Autodesk Inventor part; units mm, degrees
ref_plane "YZ Plane" through (0, 0, 0) normal (1, 0, 0) x (0, 1, 0)
ref_plane "XZ Plane" through (0, 0, 0) normal (0, 1, 0) x (-1, 0, 0)
ref_plane "XY Plane" through (0, 0, 0) normal (0, 0, 1) x (1, 0, 0)
sketch "Esboço1" plane through (0, 0, 0) normal (1, 0, 0) x (0, 1, 0)
  line L0 (0, 0) -> (0, -144)
  line L1 (0, -144) -> (52, -144)
  line L2 (52, -144) -> (52, -122)
  line L3 (52, -122) -> (16, -122)
  line L4 (0, 0) -> (38, 0)
  line L5 (38, 0) -> (52, 0)
  line L6 (16, -122) -> (16, -26)
  line L7 (16, -26) -> (52, -26)
  line L8 (52, -26) -> (52, -16)
  line L9 (52, -16) -> (38, 0)
  dimension "d0" = 144
  dimension "d1" = 52
  dimension "d2" = 22
  dimension "d3" = 36
  dimension "d8" = 38
  dimension "d10" = 96
  dimension "d12" = 10
extrude "Extrusão1" add sketch "Esboço1" against normal blind 64
sketch "Esboço2" plane through (0, 0, -144) normal (0, 0, -1) x (-1, 0, 0)
  line L0 (0, 0) -> (16, 0)
  line L1 (0, 0) -> (64, 0)
  line L2 (16, 0) -> (16, 7)
  line L3 (16, 7) -> (24, 7)
  line L4 (24, 7) -> (24, 16)
  line L5 (24, 16) -> (40, 16)
  line L6 (0, 16) -> (64, 16)
  line L7 (40, 16) -> (40, 7)
  line L8 (40, 7) -> (48, 7)
  line L9 (48, 7) -> (48, 0)
  dimension "d15" = 16
  dimension "d16" = 7
  dimension "d20" = 16
  dimension "d21" = 9
  dimension "d22" = 8
extrude "Extrusão2" cut sketch "Esboço2" against normal blind 144
sketch "Esboço3" plane through (0, 0, -144) normal (0, 0, -1) x (-1, 0, 0)
  point P0 (0, 0)
sketch "Esboço5" plane through (0, 0, -144) normal (0, 0, -1) x (-1, 0, 0)
  line L0 (48, 0) -> (64, 0)
  line L1 (0, 52) -> (64, 52)
  line L2 (64, 52) -> (64, 0)
  line L3 (40, 16) -> (64, 16)
  line L4 (24, 16) -> (40, 16)
  circle A0 centre (32, 36) radius 16
  line L5 (46.3807, 43.0139) -> (59.5563, 16)
  line L6 (17.6193, 43.0139) -> (4.4437, 16)
  line L7 (0, 0) -> (0, 52)
  line L8 (0, 0) -> (0, 16)
  line L9 (0, 16) -> (4.4437, 16)
  line L10 (0, 16) -> (24, 16)
  line L11 (59.5563, 16) -> (64, 16)
  line L12 (64, 16) -> (64, 0)
  point P0 (32, 52)
extrude "Extrusão3" cut sketch "Esboço5" against normal blind 22 contours L1 A0 L6 L9 L7 | L1 L2 L3 L5 A0
sketch "Esboço6" plane through (0, 0, -144) normal (0, 0, -1) x (-1, 0, 0)
  line L0 (24, 16) -> (40, 16)
  line L1 (32, 16) -> (32, 36)
  point P0 (0, 0)
  dimension "d49" = 20
hole "Furo1" at (-32, 36, -144) direction (0, 0, 1) diameter 13.835 depth 22
sketch "Esboço7" plane through (-64, 0, -144) normal (0, -1, 0) x (1, 0, 0)
  line L0 (0, 144) -> (0, 128)
  line L1 (10, 108) -> (10, 36)
  line L2 (54, 108) -> (54, 36)
  point P0 (64, 144)
  dimension "d59" = 72
  dimension "d61" = 72
hole "Furo2" at (-10, 0, -36) at (-10, 0, -108) at (-54, 0, -108) at (-54, 0, -36) direction (0, 1, 0) diameter 4.917 depth 12 tip angle 118
properties part number "morsa_body" material "Iron, Cast"
Geometry: final body of the model. Coordinates: model frame, mm. A direction names the side the tool comes from. Coordinates: 2 decimals unless noted, no trailing zeros. Order: outer loops, then holes, each group sorted by start corner. A loop starts at its lowest first (then second) coordinate and runs counter-clockwise, first axis right, second up. Notation, with made-up numbers: M 86.25,60 L 107.25,60 A19 cw 107.25,92 Z; hole C 28.5,38 d6. An arc over 180 degrees is marked long. Answer in a Markdown table with one row per item. Add a question column.
Q1. Contact query for flat-ended pins moving along their axis: P1, Ø12.5, axis at x = -32, y = 36, coming from the -Z side; P2, Ø2, axis at x = -17, z = -67, coming from the +Y side; P3, Ø4, axis at x = -20, z = -82, coming from the -Y side. Output: stop coordinate, or through.
Q2. Section query A-A on y = 5. Return the cut outline in (x, z), and give its area (3 significant figures).
Q3. Line query: L1, parallel to X at y = 7.75, z = -36; L2, parallel to Z at x = -10, y = 7; L3, parallel to Z at x = -32.5, y = 23. Output: solid intervals per line, ascending.
Q4. Mould query, pull axis Z, two halves, no side actions, for faces 6 (the flat face through (-40, 12, -73)), 7 (the cylindrical face through (-53.06, 6.08, -110.27)), 8 (the flat face through (-32, 45, -8)). Classes: released by +Z, released by -Z, zero draft, split by the parting line, or undercut.
Q5. Reachability of faces 1 (the cylindrical face through (-10.738, 6.084, -110.345)), 2 (the flat face through (-11.124, 29.696, -133.154)), 3 (the flat face through (-8, 0, -71)), 4 (the flat face through (-52.876, 29.696, -133.154)), 5 (the flat face through (-48, 4, -73)) from +Z, -Z, +X, -X, +Y, -Y: full face, straight path, thin tool, end or side. Return the list, or none.
Q6. Section query B-B on z = -60.5. Return the cut outline in (x, y).
Q7. Section query C-C on x = -32. Return the cut outline in (y, z).
Q8. Section query D-D on z = -125. Return the cut outline in (x, y) (1 decimal).
Completed:
| question | item | result |
|---|---|---|
| 1 | P1 | stops at z = -26 |
| 1 | P2 | stops at y = 16 |
| 1 | P3 | stops at y = 7 |
| 2 | outline | M -64,-144 L -48,-144 L -48,0 L -64,0 Z; M -16,-144 L 0,-144 L 0,0 L -16,0 Z; hole C -54,-108 d4.92; hole C -54,-36 d4.92; hole C -10,-108 d4.92; hole C -10,-36 d4.92 |
| 2 | area | 4,530 mm2 |
| 3 | L1 | x = -64 to -56.46, -51.54 to -40, -24 to -12.46, -7.54 to 0 |
| 3 | L2 | z = -144 to -110.46, -105.54 to -38.46, -33.54 to 0 |
| 3 | L3 | z = -144 to -122, -26 to 0 |
| 4 | face 6 | zero draft |
| 4 | face 7 | undercut |
| 4 | face 8 | released by +Z |
| 5 | face 1 | -Y |
| 5 | face 2 | -Z, +X, +Y |
| 5 | face 3 | +Z, -Z, +X, -X, -Y |
| 5 | face 4 | -Z, -X, +Y |
| 5 | face 5 | +Z, -Z, -Y |
| 6 | outline | M -64,0 L -48,0 L -48,7 L -40,7 L -40,16 L -64,16 Z; M -24,7 L -16,7 L -16,0 L 0,0 L 0,16 L -24,16 Z |
| 7 | outline | M 16,-144 L 29.08,-144 L 29.08,-122 L 16,-122 Z; M 16,-26 L 52,-26 L 52,-16 L 38,0 L 16,0 Z; M 42.92,-144 L 52,-144 L 52,-122 L 42.92,-122 Z |
| 8 | outline | M -64,0 L -48,0 L -48,7 L -40,7 L -40,16 L -24,16 L -24,7 L -16,7 L -16,0 L 0,0 L 0,16 L -4.4,16 L -17.6,43 A16 ccw -46.4,43 L -59.6,16 L -64,16 Z; hole C -32,36 d13.8 |
